Here's how the part is built. I have some questions about the finished solid (model axes, mm). Face numbers are marked on the shaded views. A direction names the side the tool comes from. Give positions to 0.01 mm unless a question says otherwise; leave off trailing zeros. Loops run counter-clockwise (first coordinate to the right, second up) from the corner with the lowest first, then second, coordinate; pieces in that order, holes last.
Q1. We'd pull the mould along X, two halves only. Please class the marked faces 1, 2, 3 and 4: +X half, -X half, draft (parallel to the pull), parting line (faces both ways), or undercut.
Q2. If we section it at C-C (x = 5.5): Please give me the cut outline in (y, z), plus the area to 3 significant figures.
Q3. If we section it at D-D (y = -5): Please give me the cut outline in (x, z), plus the area to 3 significant figures.
Q4. I need wall thicknesses on line 1 (Y direction, x = -13, z = 4.3); line 2 (X direction, y = -3.25, z = 3.25); line 3 (X direction, y = -8, z = 5.5). Which ranges of each line are inside material? Lowest first, please.
Q5. For the marked faces 5, 6 and 7, which set-ups out of +Z, -Z, +X, -X, +Y, -Y let a thin tool reach every point of the face, with its end or its side?
Q6. If we section it at B-B (y = -3.5): Please give me the cut outline in (x, z).
Q7. Will these pins go through, and if not, where does the flat tip stop? P1, Ø2.5, axis at x = 2.5, y = -6.5, coming from the +Z side; P2, Ø1, axis at y = -6.5, z = 1, coming from the -X side; P3, Ø1.5, axis at x = -14.5, y = -5.5, coming from the -Z side; P4, Ø0.8, axis at y = -4, z = 0.5, coming from the -X side.
Q8. If we section it at A-A (x = -13): Please give me the cut outline in (y, z).
Autodesk Inventor part; units mm, degrees
ref_plane "YZ Plane" through (0, 0, 0) normal (1, 0, 0) x (0, 1, 0)
ref_plane "XZ Plane" through (0, 0, 0) normal (0, 1, 0) x (-1, 0, 0)
ref_plane "XY Plane" through (0, 0, 0) normal (0, 0, 1) x (1, 0, 0)
ref_plane "Work Plane1" through (0, -9.3006, 0) normal (0, -1, 0) x (1, 0, 0)
sketch "Sketch1" plane through (0, -9.3006, 0) normal (0, -1, 0) x (1, 0, 0)
  line L0 (8, -4.5373) -> (-18, -4.5373)
  line L1 (8, 0) -> (8, -4.5373)
  line L2 (8, 0) -> (-18, 0)
  line L3 (-18, -4.5373) -> (-18, 0)
  line L4 (-18, 6.1006) -> (8, 6.1006)
  line L5 (8, 6.1006) -> (8, 1.1006)
  line L6 (8, 1.1006) -> (-18, 1.1006)
  line L7 (-18, 1.1006) -> (-18, 6.1006)
  line L8 (-8.5, 0.1006) -> (-1.5, 0.1006)
  line L9 (-1.5, 0.1006) -> (-1.5, 1.1006)
  line L10 (-1.5, 1.1006) -> (-8.5, 1.1006)
  line L11 (-8.5, 1.1006) -> (-8.5, 0.1006)
  line L12 (-8.5, 0.1006) -> (-1.5, 1.1006) construction
  line L13 (-1.5, 0.1006) -> (-8.5, 1.1006) construction
  point P0 (0, 0)
  point P1 (-5, 0.6006)
  dimension "d0" = 5
  dimension "d1" = 7
  dimension "d2" = 1
  dimension "d3" = 0
extrude "Extrusion1" add sketch "Sketch1" against normal blind 10 contours L4 L5 L6 L7 | L6 L9 L8 L11
sketch "Sketch2" plane through (-18, -9.3006, 6.1006) normal (0, 0, 1) x (1, 0, 0)
  circle A0 centre (5, 4.6503) radius 3.95
  circle A1 centre (21, 4.6503) radius 3.95
  point P0 (18, 9.3006)
extrude "Extrusion2" cut sketch "Sketch2" against normal blind 4
sketch "Sketch3" plane through (8, -9.3006, 6.1006) normal (1, 0, 0) x (0, 0, -1)
  line L0 (6, 0) -> (5, 0)
  line L1 (6, 0) -> (6, 10)
  line L2 (5, 10) -> (6, 10)
  line L3 (5, 0) -> (5, 10) construction
  line L4 (5, 0) -> (6, 5)
  line L5 (6, 0) -> (6, 10)
  line L6 (5, 0) -> (5, 10) construction
  line L7 (5, 10) -> (6, 5)
  point P0 (6.1006, 9.3006)
extrude "Extrusion3" cut sketch "Sketch3" against normal through all
properties part number "20_Cube_Insert_Felxuremanipulator_zonly_fiberlid"
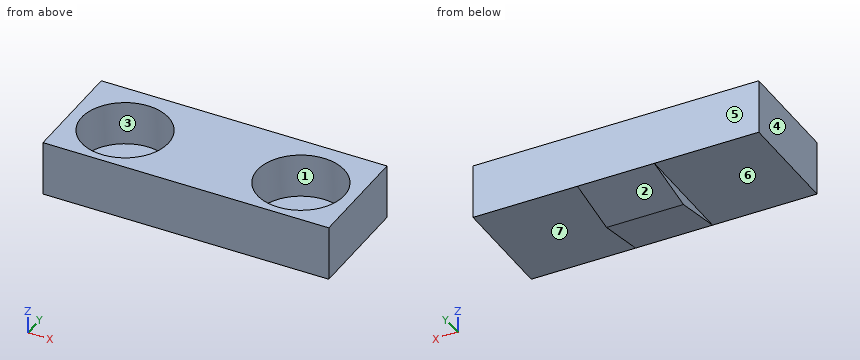
Check sheet entries:
1. face 1: undercut
1. face 2: draft
1. face 3: undercut
1. face 4: -X half
2. outline: (-9.3, 1.1) - (0.7, 1.1) - (0.7, 6.1) - (-1.59, 6.1) - (-1.59, 2.1) - (-7.71, 2.1) - (-7.71, 6.1) - (-9.3, 6.1) - close
2. area: 25.5 mm2
3. outline: (-18, 1.1) - (-8.5, 1.1) - (-8.5, 0.24) - (-1.5, 0.24) - (-1.5, 1.1) - (8, 1.1) - (8, 6.1) - (6.93, 6.1) - (6.93, 2.1) - (-0.93, 2.1) - (-0.93, 6.1) - (-9.07, 6.1) - (-9.07, 2.1) - (-16.93, 2.1) - (-16.93, 6.1) - (-18, 6.1) - close
3. area: 73.1 mm2
4. line 1: y = -9.3 to -8.6, -0.7 to 0.7
4. line 2: x = -18 to -16.69, -9.31 to -0.69, 6.69 to 8
4. line 3: x = -18 to -15.09, -10.91 to 0.91, 5.09 to 8
5. face 5: +Z, -Z, +X, -X, +Y
5. face 6: -Z, -X, +Y, -Y
5. face 7: -Z, +X, +Y, -Y
6. outline: (-18, 1.1) - (-8.5, 1.1) - (-8.5, 0.26) - (-1.5, 0.26) - (-1.5, 1.1) - (8, 1.1) - (8, 6.1) - (6.78, 6.1) - (6.78, 2.1) - (-0.78, 2.1) - (-0.78, 6.1) - (-9.22, 6.1) - (-9.22, 2.1) - (-16.78, 2.1) - (-16.78, 6.1) - (-18, 6.1) - close
7. P1: stops at z = 2.1
7. P2: stops at x = -18
7. P3: stops at z = 1.1
7. P4: stops at x = -8.5
8. outline: (-9.3, 1.1) - (0.7, 1.1) - (0.7, 6.1) - (-0.7, 6.1) - (-0.7, 2.1) - (-8.6, 2.1) - (-8.6, 6.1) - (-9.3, 6.1) - close
